Geometry: final body of the model. Coordinates: model frame, mm. Give positions to 0.01 mm unless a question says otherwise; leave off trailing zeros. Write each loop counter-clockwise with the first axis right and the second up, starting at its lowest first coordinate (ties: lowest second). Pieces come first, ordered by that corner, then holes. Notation, with made-up numbers: (-3.75, 58.5) -> (43.25, 58.5) arc R18 cw to (43.25, 66.5) -> close; hole circle Ø7 at (-16.75, 31.25). An arc over 180 degrees is marked (long way). Answer in a Markdown table with one row per item. Add a question column.
Item 1: Section query D-D on y = -0.2. Output: boundary loops of the cut face in (x, z), plus the area to 3 significant figures.
Item 2: Section query A-A on x = 15.5. Output: boundary loops of the cut face in (y, z), plus the area to 3 significant figures.
Item 3: Material intervals for probe 1 along Z at (x, y) = (31, -0.6); probe 2 along X at (y, z) = (-0.2, -1); probe 3 along Z at (x, y) = (16, -0.35), sorted ascending. Write a range as from..to.
Item 4: Section query C-C on x = 0. Output: boundary loops of the cut face in (y, z).
Item 5: Section query B-B on z = 15.5. Output: boundary loops of the cut face in (x, y).
```python
from build123d import *

# Parameters (mm, degrees)
F0_W     = 42
F0_H     = 42
F0_R     = 1.5
F0_R_2   = 11
F1_DEPTH = 1


with BuildPart() as f1:
    # F0 (on Front) → F1 (new body)
    with BuildSketch(Plane.XZ):
        with Locations((15.5, 15.5)):
            Rectangle(F0_W, F0_H)
        Circle(F0_R, mode=Mode.SUBTRACT)
        with Locations((31, 0)):
            Circle(F0_R, mode=Mode.SUBTRACT)
        with Locations((0, 31)):
            Circle(F0_R, mode=Mode.SUBTRACT)
        with Locations((15.5, 15.5)):
            Circle(F0_R_2, mode=Mode.SUBTRACT)
        with Locations((31, 31)):
            Circle(F0_R, mode=Mode.SUBTRACT)
    extrude(amount=F1_DEPTH)


solid = f1.part
```
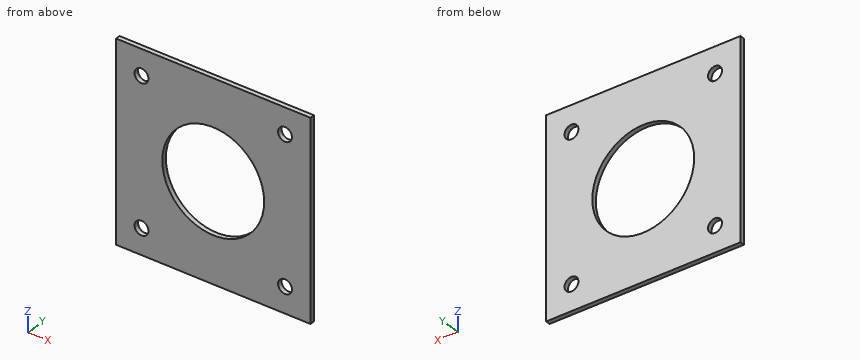
Findings below:
| question | item | result |
|---|---|---|
| 1 | outline | (-5.5, -5.5) -> (36.5, -5.5) -> (36.5, 36.5) -> (-5.5, 36.5) -> close; hole circle Ø3 at (0, 0); hole circle Ø3 at (0, 31); hole circle Ø22 at (15.5, 15.5); hole circle Ø3 at (31, 0); hole circle Ø3 at (31, 31) |
| 1 | area | 1,360 mm^2 |
| 2 | outline | (-1, -5.5) -> (0, -5.5) -> (0, 4.5) -> (-1, 4.5) -> close; (-1, 26.5) -> (0, 26.5) -> (0, 36.5) -> (-1, 36.5) -> close |
| 2 | area | 20.0 mm^2 |
| 3 | probe 1 | z = -5.5..-1.5, 1.5..29.5, 32.5..36.5 |
| 3 | probe 2 | x = -5.5..-1.12, 1.12..29.88, 32.12..36.5 |
| 3 | probe 3 | z = -5.5..4.51, 26.49..36.5 |
| 4 | outline | (-1, -5.5) -> (0, -5.5) -> (0, -1.5) -> (-1, -1.5) -> close; (-1, 1.5) -> (0, 1.5) -> (0, 29.5) -> (-1, 29.5) -> close; (-1, 32.5) -> (0, 32.5) -> (0, 36.5) -> (-1, 36.5) -> close |
| 5 | outline | (-5.5, -1) -> (4.5, -1) -> (4.5, 0) -> (-5.5, 0) -> close; (26.5, -1) -> (36.5, -1) -> (36.5, 0) -> (26.5, 0) -> close |
